from build123d import *

# Parameters (mm, degrees)
F1_DEPTH  = 10
F2_W      = 86
F2_H      = 57.5
F3_DEPTH  = 2
F5_DEPTH  = 60.001
F7_DEPTH  = 0.5
F9_DEPTH  = 0.5
F10_R     = 0.5
F11_DEPTH = 12.001
F13_DEPTH = 3


with BuildPart() as f1:
    # F0 (on Top) → F1 (new body)
    with BuildSketch(Plane.XY):
        Polygon((-58, -30), (58, -30), (58, 30), (30, 30), (30, -27.5), (-56, -27.5), (-56, 30), (-58, 30), align=None)
        with BuildLine():
            ThreePointArc((31, 15), (43.5, 27.5), (56, 15))
            Line((56, 15), (56, -15))
            ThreePointArc((56, -15), (43.5, -27.5), (31, -15))
            Line((31, -15), (31, 15))
        make_face(mode=Mode.SUBTRACT)
    extrude(amount=F1_DEPTH)

    # F2 (on face) → F3 (join)
    with BuildSketch(Plane(origin=(0, 0, 0), x_dir=(1, 0, 0), z_dir=(0, 0, -1))):
        with Locations((-13, -1.25)):
            Rectangle(F2_W, F2_H)
        Polygon((30, -30), (58, -30), (58, 30), (-58, 30), (-58, -30), (-56, -30), (-56, 27.5), (30, 27.5), align=None)
        with BuildLine():
            Line((56, 15), (56, -15))
            ThreePointArc((56, -15), (43.5, -27.5), (31, -15))
            Line((31, -15), (31, 15))
            ThreePointArc((31, 15), (43.5, 27.5), (56, 15))
        make_face(mode=Mode.SUBTRACT)
        with BuildLine():
            ThreePointArc((31, -15), (43.5, -27.5), (56, -15))
            Line((56, -15), (56, 15))
            ThreePointArc((56, 15), (43.5, 27.5), (31, 15))
            Line((31, 15), (31, -15))
        make_face()
    extrude(amount=F3_DEPTH)

    # F4 (on face) → F5 (cut, through all)
    with BuildSketch(Plane.XZ.offset(30)):
        Polygon((8.1389684882, 10), (-26, 10), (-21.1587326229, 0), (3.1389684882, 0), align=None)
    extrude(amount=-F5_DEPTH, mode=Mode.SUBTRACT)

    # F6 (on face) → F7 (join)
    with BuildSketch(Plane.XY.offset(10)):
        Polygon((-56, -27.5), (-26, -27.5), (-56, -17.5), align=None)
    extrude(amount=-F7_DEPTH)

    # F8 (on face) → F9 (join)
    with BuildSketch(Plane.XY.offset(10)):
        Polygon((30, -17.5), (8.1389684882, -27.5), (30, -27.5), align=None)
    extrude(amount=-F9_DEPTH)

    # F10 (on face) → F11 (cut, through all)
    with BuildSketch(Plane(origin=(0, 0, -2), x_dir=(1, 0, 0), z_dir=(0, 0, -1))):
        with Locations((43.5, 15)):
            Circle(F10_R)
    extrude(amount=-F11_DEPTH, mode=Mode.SUBTRACT)

    # F12 (on face) → F13 (cut)
    with BuildSketch(Plane(origin=(30, 0, 0), x_dir=(0, -1, 0), z_dir=(-1, 0, 0))):
        Polygon((15.0695058703, 10), (-14.9304941297, 10), (-10, 0), (10, 0), align=None)
    extrude(amount=-F13_DEPTH, mode=Mode.SUBTRACT)


solid = f1.part
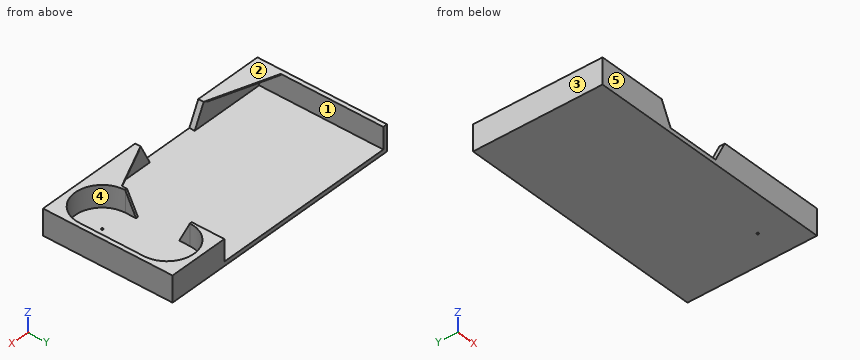
Read the model definition and answer for the solid it produces. Units are mm, in the model's axes. Face numbers are marked on the shaded views. A direction names the side the tool comes from. Give positions to 0.01 mm unless a question says otherwise; leave off trailing zeros. Write each loop counter-clockwise with the first axis right and the second up, starting at its lowest first coordinate (ties: lowest second). Pieces come first, ordered by that corner, then holes. Notation, with made-up numbers: (57, 87) - (116, 87) arc R34 ccw to (116, 122) - close; hole circle Ø11 at (-34, -20.5). An arc over 180 degrees is marked (long way). Answer in a Markdown table with one row per item. Add a question column.
Item 1: Section B-B, the plane x = -45 is taken. Write down the section's boundary in (y, z), and give its area (3 significant figures).
Item 2: A tool of negligible diameter and unlimited length cuts with its end or side. For the marked faces 1 and 2, from which of +Z, -Z, +X, -X, +Y, -Y can it reach the whole face along a straight path? Write none if from no direction.
Item 3: Section C-C, the plane y = 11.5 is taken. Write down the section's boundary in (x, z).
Item 4: A flat-ended cylindrical pin translates along its axis: P1, Ø10, axis at x = 25, y = -3, coming from the +Z side. Find the tip coordinate at first contact, or state that the pin passes through.
Item 5: Determine the mould class of the marked faces 3, 4 and 5 for opening direction X: pulls with the +X half, pulls with the -X half, needs draft (parallel to the pull), parting line crosses it, or undercut.
Item 6: Find the intervals of material crossed by L1, parallel to X at y = -12, z = 0.75; L2, parallel to X at y = -15, z = -0.5; L3, parallel to Y at x = 43.5, z = -1, in increasing order.
Item 7: Section A-A, the plane z = 3.5 is taken. Write down the section's boundary in (x, y).
Item 8: Section D-D, the plane x = 2 is taken. Write down the section's boundary in (y, z), and give its area (3 significant figures).
Recorded:
| question | item | result |
|---|---|---|
| 1 | outline | (-30, -2) - (30, -2) - (30, 0) - (-27.5, 0) - (-27.5, 9.5) - (-21.17, 9.5) - (-21.17, 10) - (-30, 10) - close |
| 1 | area | 148 mm2 |
| 2 | face 1 | +Y |
| 2 | face 2 | +Z, +X, -X, +Y, -Y |
| 3 | outline | (-58, -2) - (58, -2) - (58, 10) - (56, 10) - (56, 0) - (31, 0) - (31, 3.04) - (30, 3.04) - (30, 0) - (-56, 0) - (-56, 10) - (-58, 10) - close |
| 4 | P1 | stops at z = 0 |
| 5 | face 3 | pulls with the -X half |
| 5 | face 4 | undercut |
| 5 | face 5 | needs draft |
| 6 | L1 | x = -58 to -56, 30 to 31, 56 to 58 |
| 6 | L2 | x = -58 to 43, 44 to 58 |
| 6 | L3 | y = -30 to -15.5, -14.5 to 30 |
| 7 | outline | (-58, -30) - (-22.85, -30) - (-22.85, -27.5) - (-56, -27.5) - (-56, 30) - (-58, 30) - close; (4.89, -30) - (58, -30) - (58, 30) - (30, 30) - (30, 11.73) - (31, 11.73) - (31, 15) arc R12.5 cw to (56, 15) - (56, -15) arc R12.5 cw to (31, -15) - (31, -11.77) - (30, -11.77) - (30, -27.5) - (4.89, -27.5) - close |
| 8 | outline | (-30, -2) - (30, -2) - (30, 0) - (-30, 0) - close |
| 8 | area | 120 mm2 |
